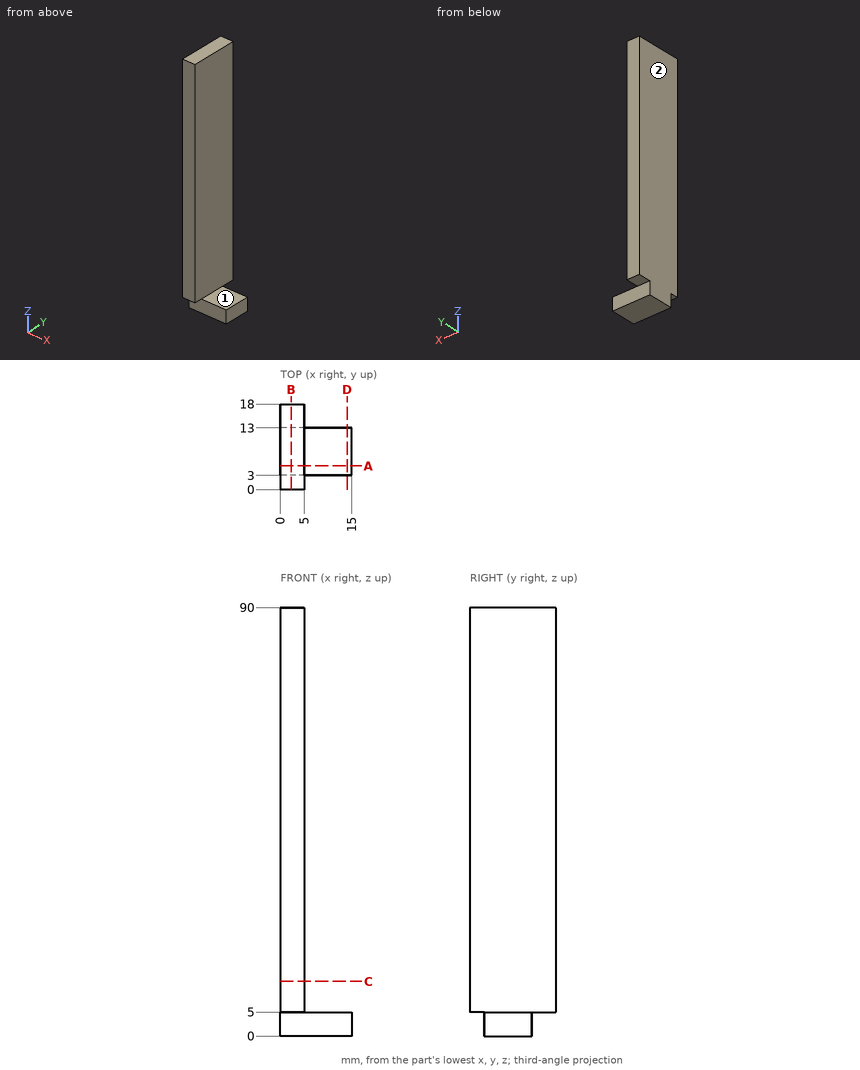
Print and shaded views of the part. All mm, measured from the part's lowest x, y and z. A direction names the side the tool comes from. Coordinates: 2 decimals unless noted, no trailing zeros. Order: outer loops, then holes, each group sorted by start corner. A loop starts at its lowest first (then second) coordinate and runs counter-clockwise, first axis right, second up. Notation, with made-up numbers: (7.5, 25) -> (49.5, 25) arc R15 cw to (49.5, 36) -> close; hole circle Ø3 at (67, -22.5). An arc over 180 degrees is marked (long way). Answer as a JSON object with one key per item and string values. Group by question number.
1) Drill centre lines: L1, parallel to Z at x = 6.5, y = 8; L2, parallel to Z at x = 3, y = 16. Where is each one in solid material? Low to high.
2) Flat gauge pins, fed straight in: pin 1 (8 mm diameter, centred on x = 10.5, y = 8.5, fed in from +Z); pin 2 (3 mm diameter, centred on y = 13, z = 10.5, fed in from -X); pin 3 (2.5 mm diameter, centred on x = 3, y = 1.5, fed in from -Z); pin 4 (8 mm diameter, centred on x = 11, z = 40.5, fed in from -Y). Where does each tip first touch, or does it go through?
3) Cut at A-A, the plane y = 5. Write the cut outline in (x, z).
4) Which spindle directions (+Z, -Z, +X, -X, +Y, -Y) get a long thin tool onto all of the face, cutting with end or side? Do the marked faces 1 and 2. Say none if no direction does.
5) Cut at B-B, the plane x = 2.25. Write the cut outline in (y, z).
6) Cut at C-C, the plane z = 11.5. Write the cut outline in (x, y).
7) Cut at D-D, the plane x = 14. Write the cut outline in (y, z).
Check values:
{
 "1": {"L1": "z = 0 to 5", "L2": "z = 5 to 90"},
 "2": {"pin 1": "stops at z = 5", "pin 2": "stops at x = 0", "pin 3": "stops at z = 5", "pin 4": "passes through"},
 "3": {"outline": "(0, 0) -> (15, 0) -> (15, 5) -> (5, 5) -> (5, 90) -> (0, 90) -> close"},
 "4": {"face 1": "+Z, +X, +Y, -Y", "face 2": "+Z, -Z, -X, +Y, -Y"},
 "5": {"outline": "(0, 5) -> (3, 5) -> (3, 0) -> (13, 0) -> (13, 5) -> (18, 5) -> (18, 90) -> (0, 90) -> close"},
 "6": {"outline": "(0, 0) -> (5, 0) -> (5, 18) -> (0, 18) -> close"},
 "7": {"outline": "(3, 0) -> (13, 0) -> (13, 5) -> (3, 5) -> close"}
}
